Build history of the part. All positions in model axes, mm. Face numbers are marked on the shaded views. A direction names the side the tool comes from. Round coordinates to 2 decimals unless told otherwise and drop trailing zeros. Order: outer loops, then holes, each group sorted by start corner. A loop starts at its lowest first (then second) coordinate and runs counter-clockwise, first axis right, second up. Notation, with made-up numbers: (51, 31.25) -> (82, 31.25) arc R26 ccw to (82, 47.25) -> close; hole circle Ø3 at (-9, -16). An arc over 180 degrees is marked (long way). Use a Markdown table: item, result. Add a question column.
Item 1: Two-plate mould, pull along Z, no slides. Class the marked faces 4, 5 and 6: released by +Z, released by -Z, zero draft, split by the parting line, or undercut.
Item 2: Slice it at B-B, the plane x = -20.5. Give the cut face in (y, z), plus the area to 3 significant figures.
Item 3: Slice it at D-D, the plane y = 3. Give the cut face in (x, z), plus the area to 3 significant figures.
Item 4: Probe L1, parallel to X at y = 6, z = -32; L2, parallel to Z at x = 41, y = 14; L3, parallel to Z at x = -24, y = 4.5. List the from-to ranges inside material, lowest first.
Item 5: Slice it at A-A, the plane y = 15.5. Give the cut face in (x, z).
Item 6: 3-axis set-ups, long thin cutter, end or side, ignore diameter. For the marked faces 1, 2 and 3: which of +Z, -Z, +X, -X, +Y, -Y reach the whole face in a straight line?
Item 7: Pin check, flat tips, straight feed: pin 1 (5 mm diameter, centred on x = -2.5, z = 17, fed in from +Y); pin 2 (2 mm diameter, centred on x = -6, y = 30.5, fed in from -Z); pin 3 (8 mm diameter, centred on x = -4, z = 2, fed in from -Y). Stop position of each tip, or through.
Item 8: Slice it at C-C, the plane z = -24.5. Give the cut face in (x, y).
from build123d import *

# Parameters (mm, degrees)
SKETCH_1_W          = 120.704131687
SKETCH_1_H          = 73.359986831
EXTRUDE_1_DEPTH     = 32
FILLET_4_R          = 5
SKETCH_2_W          = 103.308329398
SKETCH_2_H          = 57.020562217
EXTRUDE_2_DEPTH     = 1
SKETCH_3_W          = 106.896586693
SKETCH_3_H          = 59.364518817
CUT_EXTRUDE_1_DEPTH = 2
EXTRUDE_4_DEPTH     = 2
SKETCH_6_W          = 107.275121148
SKETCH_6_H          = 59.528469182
CUT_EXTRUDE_2_DEPTH = 26


with BuildPart() as part:
    # 草图1 → 凸台-拉伸1 (new body)
    with BuildSketch(Plane(origin=(0, 0, 0), x_dir=(1, 0, 0), z_dir=(0, 1, 0))):
        with Locations((-12.539167079, 5.976612345)):
            Rectangle(SKETCH_1_W, SKETCH_1_H)
    extrude(amount=EXTRUDE_1_DEPTH)

    # 圆角4
    fillet_4_edges = [part.edges().sort_by_distance(p)[0] for p in [
        (-12.539167078, 32, -42.656605761),
        (-72.891232922, 32, -5.976612346),
        (-12.539167078, 32, 30.70338107),
        (-72.891232922, 0, -5.976612346),
        (-12.539167078, 0, -42.656605761),
        (47.812898765, 0, -5.976612346),
        (-12.539167078, 0, 30.70338107),
        (-72.891232922, 16, 30.70338107),
        (-72.891232922, 16, -42.656605761),
        (47.812898765, 16, -42.656605761),
        (47.812898765, 16, 30.70338107),
        (47.812898765, 32, -5.976612346),
    ]]
    fillet(fillet_4_edges, radius=FILLET_4_R)

    # 草图2 → 凸台-拉伸2 (add)
    with BuildSketch(Plane(origin=(0, 32, 0), x_dir=(1, 0, 0), z_dir=(0, 1, 0))):
        with Locations((-12.689078598, 6.094786595)):
            Rectangle(SKETCH_2_W, SKETCH_2_H)
    extrude(amount=-EXTRUDE_2_DEPTH)

    # 草图3 → 切除-拉伸1 (cut)
    with BuildSketch(Plane(origin=(0, 32, 0), x_dir=(1, 0, 0), z_dir=(0, 1, 0))):
        with Locations((-12.5895853, 5.984959014)):
            Rectangle(SKETCH_3_W, SKETCH_3_H)
    extrude(amount=-CUT_EXTRUDE_1_DEPTH, mode=Mode.SUBTRACT)

    # 草图5 → 凸台-拉伸4 (add)
    with BuildSketch(Plane(origin=(0, 30, 0), x_dir=(1, 0, 0), z_dir=(0, 1, 0))):
        with BuildLine():
            Line((-35.374881663, 22.419896032), (11.907439302, 22.419896032))
            ThreePointArc((11.907439302, 22.419896032), (26.657556761, 7.669778573), (11.907439302, -7.080338886))
            Line((11.907439302, -7.080338886), (-35.374881663, -7.080338886))
            ThreePointArc((-35.374881663, -7.080338886), (-50.124999122, 7.669778573), (-35.374881663, 22.419896032))
        make_face()
    extrude(amount=EXTRUDE_4_DEPTH)

    # 草图6 → 切除-拉伸2 (cut)
    with BuildSketch(Plane.XZ):
        with Locations((-12.51647611, -5.961067915)):
            Rectangle(SKETCH_6_W, SKETCH_6_H)
    extrude(amount=-CUT_EXTRUDE_2_DEPTH, mode=Mode.SUBTRACT)


solid = part.part
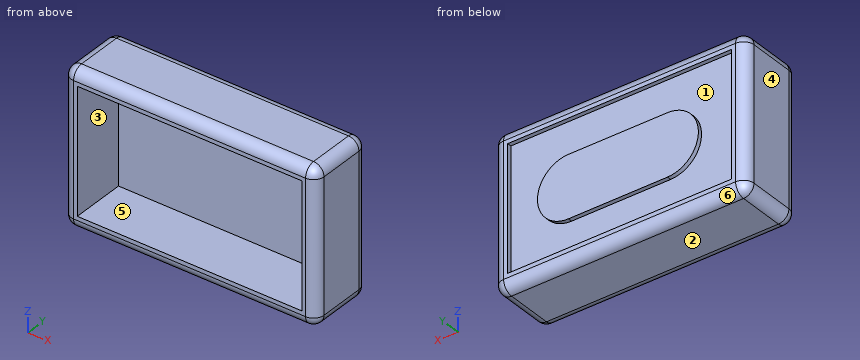
Check sheet entries:
| question | item | result |
|---|---|---|
| 1 | face 4 | zero draft |
| 1 | face 5 | undercut |
| 1 | face 6 | released by -Z |
| 2 | outline | (0, -37.66) arc R5 ccw to (5, -42.66) -> (27, -42.66) arc R5 ccw to (32, -37.66) -> (32, -35.67) -> (30, -35.67) -> (30, -22.42) -> (32, -22.42) -> (32, 7.08) -> (30, 7.08) -> (30, 23.7) -> (32, 23.7) -> (32, 25.7) arc R5 ccw to (27, 30.7) -> (5, 30.7) arc R5 ccw to (0, 25.7) -> (0, 23.8) -> (26, 23.8) -> (26, -35.73) -> (0, -35.73) -> close |
| 2 | area | 719 mm2 |
| 3 | outline | (-72.47, -37.66) arc R4.58 ccw to (-67.89, -42.24) -> (42.81, -42.24) arc R4.58 ccw to (47.4, -37.66) -> (47.4, 25.7) arc R4.58 ccw to (42.81, 30.29) -> (-67.89, 30.29) arc R4.58 ccw to (-72.47, 25.7) -> close; hole (-66.15, -35.73) -> (41.12, -35.73) -> (41.12, 23.8) -> (-66.15, 23.8) -> close |
| 3 | area | 2,290 mm2 |
| 4 | L1 | -72.89 to -66.15, 41.12 to 47.81 |
| 4 | L2 | -42.66 to -35.73, 23.8 to 30.7 |
| 4 | L3 | -42.63 to -35.73, 23.8 to 30.68 |
| 5 | outline | (-72.89, -37.66) arc R5 ccw to (-67.89, -42.66) -> (42.81, -42.66) arc R5 ccw to (47.81, -37.66) -> (47.81, 25.7) arc R5 ccw to (42.81, 30.7) -> (-67.89, 30.7) arc R5 ccw to (-72.89, 25.7) -> close; hole (-66.15, -35.73) -> (41.12, -35.73) -> (41.12, 23.8) -> (-66.15, 23.8) -> close |
| 6 | face 1 | +Y |
| 6 | face 2 | -Z, +X, -X, +Y, -Y |
| 6 | face 3 | -Y |
| 7 | pin 1 | y = 30 |
| 7 | pin 2 | z = -41.99 |
| 7 | pin 3 | y = 26 |
| 8 | outline | (-72.89, 5) arc R5 ccw to (-67.89, 0) -> (-66.15, 0) -> (-66.15, 26) -> (41.12, 26) -> (41.12, 0) -> (42.81, 0) arc R5 ccw to (47.81, 5) -> (47.81, 27) arc R5 ccw to (42.81, 32) -> (40.86, 32) -> (40.86, 30) -> (-66.04, 30) -> (-66.04, 32) -> (-67.89, 32) arc R5 ccw to (-72.89, 27) -> close |
